Verification items for the finished model (mm, model axes). A direction names the side the tool comes from. Give positions to 0.01 mm unless a question says otherwise; leave off trailing zeros. Loops run counter-clockwise (first coordinate to the right, second up) from the corner with the lowest first, then second, coordinate; pieces in that order, holes last. Notation, with made-up numbers: (2, 32.25) -> (49, 32.25) arc R32 cw to (49, 62.25) -> close; hole circle Ø10 at (56, 83). An arc over 180 degrees is marked (long way). Use one line per item in the form item = value. Start each with the question number.
from build123d import *

# Parameters (mm, degrees)
BOSS_EXTRUDE2_DEPTH = 15
SKETCH2_R           = 4
CUT_EXTRUDE1_DEPTH  = 20
SKETCH3_R           = 6
CUT_EXTRUDE2_DEPTH  = 2.5
CUT_EXTRUDE3_START  = -2.5
SKETCH4_R           = 6
CUT_EXTRUDE3_DEPTH  = 2.5
FILLET1_R           = 7.5
BOSS_EXTRUDE3_DEPTH = 3
SKETCH6_W           = 10
SKETCH6_H           = 30
BOSS_EXTRUDE4_DEPTH = 3
CUT_EXTRUDE4_DEPTH  = 10
SKETCH8_R           = 4
BOSS_EXTRUDE6_DEPTH = 5
REVOLVE3_ANGLE      = 180
CUT_EXTRUDE6_DEPTH  = 15


with BuildPart() as part:
    # Sketch1 → Boss-Extrude2 (new body)
    with BuildSketch(Plane.XY):
        Polygon((4.00158439, 29.571674002), (4.00158439, 14.571674002), (-5.99841561, 14.571674002), (-5.99841561, 29.571674002), (-10.99841561, 29.571674002), (-10.99841561, -40.428325998), (9.00158439, -40.428325998), (9.00158439, 29.571674002), align=None)
    extrude(amount=BOSS_EXTRUDE2_DEPTH)

    # Sketch2 → Cut-Extrude1 (cut)
    with BuildSketch(Plane.ZY.offset(10.99841561)):
        with Locations((7.5, 22.071674002)):
            Circle(SKETCH2_R)
    extrude(amount=-CUT_EXTRUDE1_DEPTH, mode=Mode.SUBTRACT)

    # Sketch3 → Cut-Extrude2 (cut)
    with BuildSketch(Plane.ZY.offset(10.99841561)):
        with Locations((7.5, 22.071674002)):
            Circle(SKETCH3_R)
    extrude(amount=-CUT_EXTRUDE2_DEPTH, mode=Mode.SUBTRACT)

    # Sketch4 → Cut-Extrude3 (cut)
    with BuildSketch(Plane(origin=(9.00158439, 0, 0), x_dir=(0, 0, -1), z_dir=(1, 0, 0)).offset(CUT_EXTRUDE3_START)):
        with Locations(Location((-7.5, 22.071674002, 0), (0, 0, 180))):
            Circle(SKETCH4_R)
    extrude(amount=CUT_EXTRUDE3_DEPTH, mode=Mode.SUBTRACT)

    # Fillet1
    fillet1_edges = [part.edges().sort_by_distance(p)[0] for p in [
        (6.50158439, 29.571674002, 0),
        (6.50158439, 29.571674002, 15),
        (-8.49841561, 29.571674002, 0),
        (-8.49841561, 29.571674002, 15),
    ]]
    fillet(fillet1_edges, radius=FILLET1_R - 0.0001)  # a hair under: the kernel refuses the full size

    # Sketch5 → Boss-Extrude3 (add)
    with BuildSketch(Plane.XY.offset(15)):
        Polygon((-5.99841561, 9.571674002), (-5.99841561, -15.428325998), (-3.99841561, -20.428325998), (2.00158439, -20.428325998), (4.00158439, -15.428325998), (4.00158439, 9.571674002), (9.00158439, 14.571674002), (9.00158439, 29.571674002), (-10.99841561, 29.571674002), (-10.99841561, 14.548804666), align=None)
    extrude(amount=BOSS_EXTRUDE3_DEPTH)

    # Sketch6 → Boss-Extrude4 (add)
    with BuildSketch(Plane.XY.offset(18)):
        with Locations((-0.99841561, 19.571674002)):
            Rectangle(SKETCH6_W, SKETCH6_H)
    extrude(amount=BOSS_EXTRUDE4_DEPTH)

    # Sketch7 → Cut-Extrude4 (cut)
    with BuildSketch(Plane.ZY.offset(5.99841561)):
        Polygon((21, 14.548804666), (18, 4.571674002), (21, 4.571674002), align=None)
    extrude(amount=-CUT_EXTRUDE4_DEPTH, mode=Mode.SUBTRACT)

    # Sketch8 → Boss-Extrude6 (add)
    with BuildSketch(Plane.XZ.offset(40.428325998)):
        with Locations(Location((-0.99841561, 7.5, 0), (0, 0, 270))):
            Circle(SKETCH8_R)
    extrude(amount=BOSS_EXTRUDE6_DEPTH)

    # Sketch9 → Revolve3 (revolve)
    with BuildSketch(Plane(origin=(0, -45.428325998, 0), x_dir=(-1, 0, 0), z_dir=(0, -1, 0))):
        with BuildLine():
            Line((0.99841561, -12.5), (0.99841561, -2.5))
            ThreePointArc((0.99841561, -2.5), (5.99841561, -7.5), (0.99841561, -12.5))
        make_face()
    revolve(axis=Axis((-0.99841561, -45.428325998, 12.5), (0, 0, 1)), revolution_arc=REVOLVE3_ANGLE)

    # Sketch10 → Cut-Extrude6 (cut)
    with BuildSketch(Plane.XY.offset(15)):
        Polygon((6.335572216, -30.967221552), (2.949498735, -40.428325998), (9.00158439, -40.428325998), (9.00158439, 4.571674002), (6.335572216, -6.092374694), align=None)
        Polygon((-8.49841561, -24.415311945), (-8.49841561, -5.428325998), (-10.99841561, 4.571674002), (-10.99841561, -40.428325998), (-4.99841561, -40.428325998), (-8.49841561, -30.967221552), align=None)
    extrude(amount=-CUT_EXTRUDE6_DEPTH, mode=Mode.SUBTRACT)


solid = part.part
Item 1: Sectioned sample at B-B, the plane y = -1. Enter the section's corners in (x, z), and give its area (3 significant figures).
Item 2: Draft check along Z on faces 4 (the cylindrical face through (5.234, 22.248, 3.504)), 5 (the flat face through (-1, 25, 21)), 6 (the flat face through (-8.498, -18, 8)). Enter one of: +Z half, -Z half, draft (parallel to the pull), parting line (faces both ways), or undercut.
Item 3: Sectioned sample at A-A, the plane x = -0.25. Enter the section's corners in (y, z), and give its area (3 significant figures).
Item 4: Material ranges on line 1 (Z direction, x = 8.25, y = 27); line 2 (Z direction, x = 5.75, y = 15); line 3 (Z direction, x = 6.25, y = 24), recorded low to high.
Item 5: Sectioned sample at D-D, the plane y = 8. Enter the section's corners in (x, z), and give its area (3 significant figures).
Item 6: Tool access check on faces 1 (the flat face through (-8.498, 18, 9)), 2 (the flat face through (3, -19, 15)), 3 (the flat face through (-9, 22, 18)). Record the directions out of +Z, -Z, +X, -X, +Y, -Y that give a thin tool (end or side, any length) a straight path to the whole face; none if there is none.
Item 7: Gauge pin test, flat ends, axial feed: pin 1 Ø4.5 at (x, y) = (-2, 23.5) entering from -Z; pin 2 Ø6.5 at (y, z) = (22.07, 7.5) entering from -X; pin 3 Ø3.5 at (y, z) = (22.5, 10) entering from +X; pin 4 Ø12 at (x, y) = (5.5, -41) entering from +Z. Record the tip position at first contact, or that the pin passes through.
Outcome:
q1.outline = (-9.61, 0) -> (7.61, 0) -> (7.61, 15) -> (4, 15) -> (4, 18) -> (-6, 18) -> (-6, 15) -> (-9.61, 15) -> close
q1.area = 288 mm^2
q2.face_4 = undercut
q2.face_5 = +Z half
q2.face_6 = draft
q3.outline = (-45.43, 2.56) -> (-45.43, 3.57) -> (-40.43, 3.57) -> (-40.43, 0) -> (14.57, 0) -> (14.57, 15) -> (29.57, 15) -> (29.57, 18) -> (34.57, 18) -> (34.57, 21) -> (14.55, 21) -> (4.57, 18) -> (-20.43, 18) -> (-20.43, 15) -> (-40.43, 15) -> (-40.43, 11.43) -> (-45.43, 11.43) -> (-45.43, 12.44) arc R4.94 ccw to start
q3.area = 1,130 mm^2
q4.line_1 = 1.85 to 4.08, 10.92 to 13.15, 15 to 18
q4.line_2 = 0 to 18
q4.line_3 = 0.25 to 4, 11 to 14.75, 15 to 18
q5.outline = (-11, 0) -> (9, 0) -> (9, 15) -> (4, 15) -> (4, 19.03) -> (-6, 19.03) -> (-6, 15) -> (-11, 15) -> close
q5.area = 340 mm^2
q6.face_1 = -X
q6.face_2 = +Z, -Y
q6.face_3 = +Z, -X, +Y, -Y
q7.pin_1 = 15
q7.pin_2 = through
q7.pin_3 = 6.5
q7.pin_4 = 15
